Part print with two shaded views. Sizes in mm from the minimum x, y, z corner. A direction names the side the tool comes from. Give positions to 0.01 mm unless a question says otherwise; leave off trailing zeros. Order: outer loops, then holes, each group sorted by start corner. A loop starts at its lowest first (then second) coordinate and runs counter-clockwise, first axis right, second up. Notation, with made-up numbers: M 68.5,82.25 L 89.5,82.25 A23 ccw 89.5,93.25 Z; hole C 41.5,67 d9. An arc over 180 degrees is marked long. Return JSON: item names as keys, results as strings. Group by question number.
1. Slice it at A-A on x = 26. List the corners of the cut face in (y, z), then the cut area to 3 significant figures.
2. Two-plate mould, pull along Y, no slides. Class the marked faces 4, 5 and 6: released by +Y, released by -Y, zero draft, split by the parting line, or undercut.
3. Pin check, flat tips, straight feed: pin 1 (12 mm diameter, centred on y = 24, z = 73, fed in from -X); pin 2 (9 mm diameter, centred on x = 13, z = 12.5, fed in from +Y); pin 3 (3 mm diameter, centred on y = 102.5, z = 60.5, fed in from +X); pin 4 (12 mm diameter, centred on x = 68, z = 68, fed in from +Y) (1 decimal). Stop position of each tip, or through.
4. Slice it at C-C on z = 12. List the corners of the cut face in (x, y), then the cut area to 3 significant figures.
5. 3-axis set-ups, long thin cutter, end or side, ignore diameter. For the marked faces 1, 2 and 3: which of +Z, -Z, +X, -X, +Y, -Y reach the whole face in a straight line?
6. Slice it at B-B on y = 93. List the corners of the cut face in (x, z).
7. Wall check: probe 1 along Z at (x, y) = (22, 103); probe 2 along Z at (x, y) = (78.5, 61.5); probe 3 along X at (y, z) = (96, 12). Give the ranges that are in metal, low to high. Write a range as [from, to].
8. Slice it at D-D on x = 90.5. List the corners of the cut face in (y, z) (1 decimal).
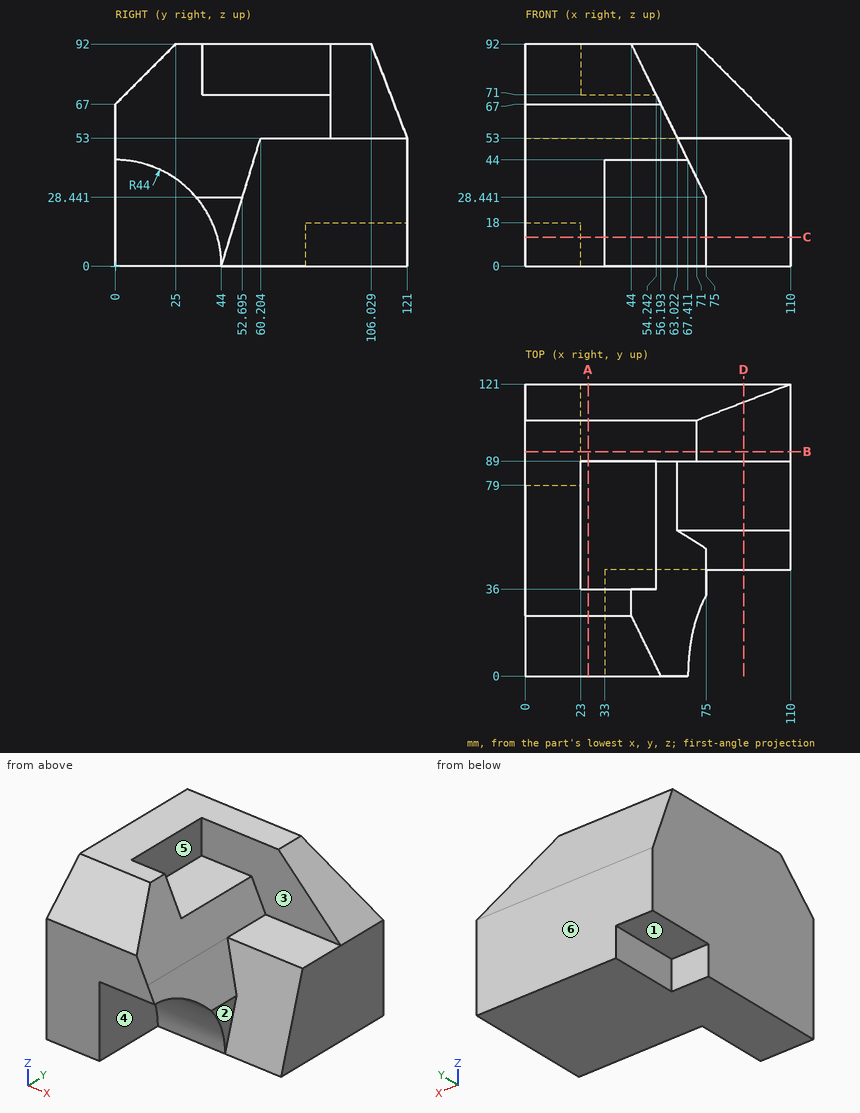
Result:
{
 "1": {"outline": "M 0,0 L 121,0 L 121,53 L 106.03,92 L 89,92 L 89,71 L 36,71 L 36,92 L 25,92 L 0,67 Z", "area": "9,410 mm2"},
 "2": {"face 4": "zero draft", "face 5": "undercut", "face 6": "released by +Y"},
 "3": {"pin 1": "stops at x = 0", "pin 2": "stops at y = 79", "pin 3": "stops at x = 104", "pin 4": "stops at y = 117.5"},
 "4": {"outline": "M 0,0 L 33,0 L 33,42.33 L 75,42.33 L 75,47.67 L 110,47.67 L 110,121 L 23,121 L 23,79 L 0,79 Z", "area": "8,900 mm2"},
 "5": {"face 1": "-Z, -X, +Y", "face 2": "+Z, +X, -Y", "face 3": "+Z, +X"},
 "6": {"outline": "M 0,18 L 23,18 L 23,0 L 110,0 L 110,53 L 71,92 L 0,92 Z"},
 "7": {"probe 1": "z = [18, 92]", "probe 2": "z = [0, 53]", "probe 3": "x = [23, 110]"},
 "8": {"outline": "M 44,0 L 121,0 L 121,53 L 113.5,72.5 L 89,72.5 L 89,53 L 60.2,53 Z"}
}
